from build123d import *

# Parameters (mm, degrees)
F1_DEPTH       = 18
F4_D           = 8
F4_DEPTH       = 21
F4_TIP         = 2.4034424761
F4_ON_F2_D     = 8
F4_ON_F2_DEPTH = 21
F4_ON_F2_TIP   = 2.4034424761


with BuildPart() as f1:
    # F0 (on Top) → F1 (new body)
    with BuildSketch(Plane.XY):
        with BuildLine():
            ThreePointArc((279.7628534604, 271.7218169814), (15.5579598443, 389.6895557819), (-257.2105231107, 293.1599338265))
            Line((-257.2105231107, 293.1599338265), (0.5571067524, 13.9541871184))
            Line((0.5571067524, 13.9541871184), (279.7628534604, 271.7218169814))
        make_face()
    extrude(amount=F1_DEPTH)

    # F4
    with Locations(Plane(origin=(-6.698540183, 7.2556469354, 0), x_dir=(0.734751965, 0.6783358681, 0), z_dir=(0.6783358681, -0.734751965, 0))):
        with Locations((110.3749609131, 9), (229.8749609131, 9)):
            Hole(F4_D / 2, depth=F4_DEPTH)
            with Locations((0, 0, -(F4_DEPTH + F4_TIP / 2))):  # 118° drill point
                Cone(0, F4_D / 2, F4_TIP, mode=Mode.SUBTRACT)

    # F4 on F2
    with Locations(Plane(origin=(7.2556469354, 6.698540183, 0), x_dir=(0.6783358681, -0.734751965, 0), z_dir=(-0.734751965, -0.6783358681, 0))):
        with Locations((-110.3749609131, 9), (-229.8749609131, 9)):
            Hole(F4_ON_F2_D / 2, depth=F4_ON_F2_DEPTH)
            with Locations((0, 0, -(F4_ON_F2_DEPTH + F4_ON_F2_TIP / 2))):  # 118° drill point
                Cone(0, F4_ON_F2_D / 2, F4_ON_F2_TIP, mode=Mode.SUBTRACT)


solid = f1.part
Input: part model. Units: mm. Frame: model coordinates. Round coordinates to 2 decimals unless told otherwise and drop trailing zeros. Order: outer loops, then holes, each group sorted by start corner. A loop starts at its lowest first (then second) coordinate and runs counter-clockwise, first axis right, second up.
1. Material intervals for line 1 (X direction, y = 179, z = 7); line 2 (X direction, y = 183, z = 12); line 3 (X direction, y = 290.5, z = 2.75), sorted ascending.
The answers:
line 1: x = -151.82 to -150.1, -139.89 to 146.7, 152.32 to 179.33
line 2: x = -155.51 to -144.56, -136.76 to 183.66
line 3: x = -254.75 to 260.21
2. Cut plane A-A, the plane y = 366. Output: boundary loops of the cut face in (x, z).
The answers:
outline: (-134.7, 0) - (134.7, 0) - (134.7, 18) - (-134.7, 18) - close
3. Pin query (flat end, axial travel): P1, Ø1, axis at x = -186.5, z = 16, coming from the -Y side; P2, Ø2, axis at x = -68.5, z = 3.5, coming from the -Y side; P3, Ø2, axis at y = 102, z = 2, coming from the -X side. Return the tip coordinate at first contact, or that it passes through.
The answers:
P1: stops at y = 216.03
P2: stops at y = 87.67
P3: stops at x = -81.65
4. Mould query, pull axis Z, two halves, no side actions, for faces 1 (the face through (19.704, 389.502, 8.874)), 2 (the face through (-138.14, 179.89, 9.18)), 3 (the face through (152.27, 168.5, 7.47)), 4 (the face through (8, 246, 18)). Classes: released by +Z, released by -Z, zero draft, split by the parting line, or undercut.
The answers:
face 1: zero draft
face 2: undercut
face 3: undercut
face 4: released by +Z
5. Cut plane B-B, the plane x = 13. Output: boundary loops of the cut face in (y, z), then the cut area to 3 significant figures.
The answers:
outline: (25.44, 0) - (389.78, 0) - (389.78, 18) - (25.44, 18) - close
area: 6,560 mm2
